Read the model definition and answer for the solid it produces. Units are mm, in the model's axes. Round coordinates to 2 decimals unless told otherwise and drop trailing zeros. Write each loop counter-clockwise with the first axis right and the second up, starting at its lowest first coordinate (ties: lowest second). Pieces come first, ordered by that corner, then holes.
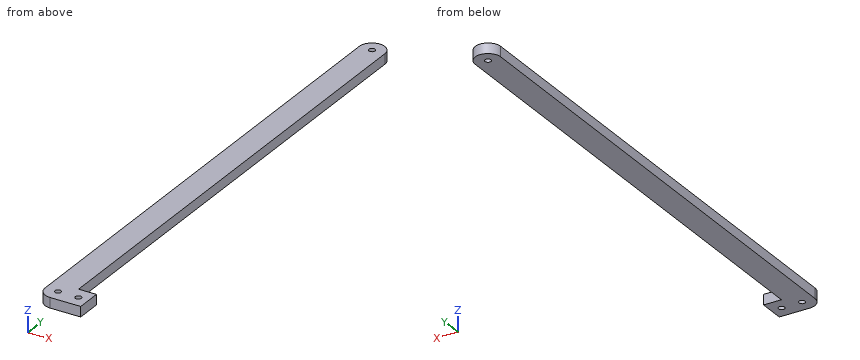
from build123d import *

# Parameters (mm, degrees)
SKETCH1_R           = 3
BOSS_EXTRUDE1_DEPTH = 10


with BuildPart() as part:
    # Sketch1 → Boss-Extrude1 (new body)
    with BuildSketch(Plane.XY):
        with BuildLine():
            Line((-12.5, 0), (-12.5, -499.599839872))
            ThreePointArc((-12.5, -499.599839872), (-8.838834765, -508.438674637), (0, -512.099839872))
            Line((0, -512.099839872), (30, -512.099839872))
            Line((30, -512.099839872), (30, -487.099839872))
            Line((30, -487.099839872), (12.5, -487.099839872))
            Line((12.5, -487.099839872), (12.5, 0))
            ThreePointArc((12.5, 0), (0, 12.5), (-12.5, 0))
        make_face()
        Circle(SKETCH1_R, mode=Mode.SUBTRACT)
        with Locations(Location((0, -499.599839872, 0), (0, 0, 180))):
            Circle(SKETCH1_R, mode=Mode.SUBTRACT)
        with Locations((20, -499.599839872)):
            Circle(SKETCH1_R, mode=Mode.SUBTRACT)
    extrude(amount=BOSS_EXTRUDE1_DEPTH)


solid = part.part
Q1. Flat-ended cylindrical pins translate along their axes: pin 1 Ø1.5 at (x, z) = (-8, 1) entering from +Y; pin 2 Ø1.5 at (x, y) = (-0.5, -227) entering from -Z; pin 3 Ø5 at (y, z) = (-304, 3.5) entering from +X; pin 4 Ø5.5 at (x, y) = (0, -499.6) entering from -Z. Find the tip coordinate at first contact, or state that the pin passes through.
Verdict:
pin 1: stops at y = 10.18
pin 2: stops at z = 0
pin 3: stops at x = 12.5
pin 4: passes through
Q2. Straight lines are drawn through the part: probe 1 along Y at (x, z) = (20, 3.25); probe 2 along Y at (x, z) = (-1, 2.5); probe 3 along X at (y, z) = (-425, 2.25). For each, find the intervals that lie inside material, in ascending order.
Verdict:
probe 1: y = -512.1 to -502.6, -496.6 to -487.1
probe 2: y = -512.06 to -502.43, -496.77 to -2.83, 2.83 to 12.46
probe 3: x = -12.5 to 12.5
Q3. Section A-A (z = 5.75) is taken. Determine the outline of the cut face in (x, y).
Verdict:
outline: (-12.5, -499.6) arc R12.5 ccw to (0, -512.1) - (30, -512.1) - (30, -487.1) - (12.5, -487.1) - (12.5, 0) arc R12.5 ccw to (-12.5, 0) - close; hole circle Ø6 at (0, -499.6); hole circle Ø6 at (0, 0); hole circle Ø6 at (20, -499.6)
Q4. Section B-B (y = -297) is taken. Determine the outline of the cut face in (x, z), then the cut area to 3 significant figures.
Verdict:
outline: (-12.5, 0) - (12.5, 0) - (12.5, 10) - (-12.5, 10) - close
area: 250 mm2
